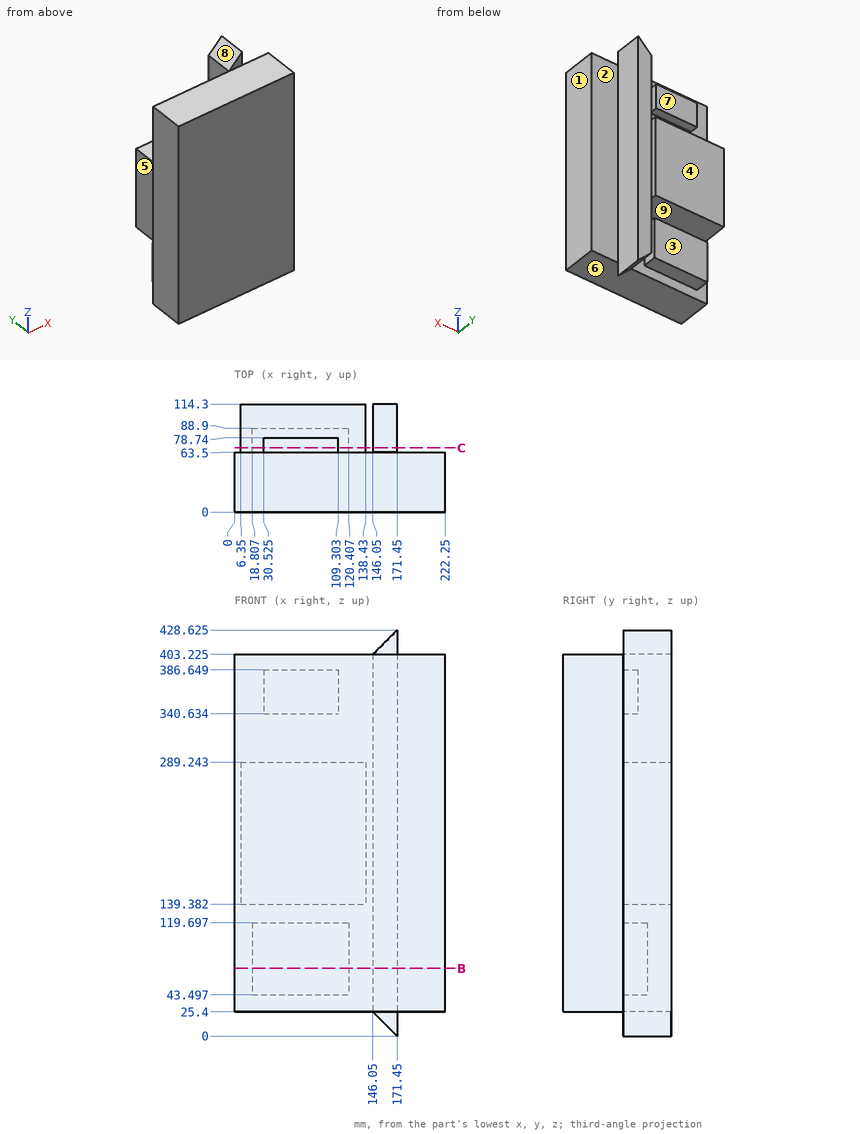
Geometry check sheet. Reference: drawing and pictorial views, mm from the part's lowest x, y, z. A direction names the side the tool comes from. Round coordinates to 2 decimals unless told otherwise and drop trailing zeros. Write each loop counter-clockwise with the first axis right and the second up, starting at its lowest first coordinate (ties: lowest second). Pieces come first, ordered by that corner, then holes. Notation, with made-up numbers: (19.5, -8.75) -> (58.5, -8.75) arc R20 cw to (58.5, 16.25) -> close; hole circle Ø1 at (46, -26). An arc over 180 degrees is marked (long way). Put each result on its own line as item: value.
1) Depth check by flat-ended pin: P1, Ø1.5, axis at x = 193, z = 345, coming from the +Y side; P2, Ø12, axis at x = 70.5, y = 74.5, coming from the +Z side; P3, Ø4.5, axis at y = 67.5, z = 365.5, coming from the -X side (1 decimal). Enter the tip coordinate at first touch or a pass-through.
Recorded:
P1: stops at y = 63.5
P2: stops at z = 386.65
P3: stops at x = 30.5
2) Cross-section at B-B, the plane z = 71.5. Enter the section's corners in (x, y).
Recorded:
outline: (0, 0) -> (222.25, 0) -> (222.25, 63.5) -> (171.45, 63.5) -> (171.45, 114.3) -> (146.05, 114.3) -> (146.05, 63.5) -> (120.41, 63.5) -> (120.41, 88.9) -> (18.81, 88.9) -> (18.81, 63.5) -> (0, 63.5) -> close
3) Cross-section at C-C, the plane y = 68. Give the number of separate pieces and of enclosed holes in the cut face, plus the area to 3 significant figures.
Recorded:
separate pieces: 4
enclosed holes: 0
area: 41,400 mm2
4) Release check for a two-part mould opening along Z. For the marked faces 6, 7, 8 and 9 record: pulls with the +Z half, pulls with the -Z half, needs draft (parallel to the pull), parting line crosses it, or undercut.
Recorded:
face 6: pulls with the -Z half
face 7: needs draft
face 8: pulls with the +Z half
face 9: undercut
5) Access from +Z, -Z, +X, -X, +Y, -Y to the whole of each face (thin tool, end or side, straight path). Record for the marked faces 1, 2, 3, 4 and 5.
Recorded:
face 1: +Z, -Z, +X, +Y, -Y
face 2: +Z, -Z, +X, +Y
face 3: -Z, -X, +Y
face 4: +Z, -Z, +X, -X, +Y
face 5: +Z, -Z, -X, +Y
6) Thickness scan on probe 1 along X at (y, z) = (86, 263); probe 2 along Z at (x, y) = (51, 67); probe 3 along Z at (x, y) = (62, 99.5). Record the ranges inside material, lowest first. Write a range as from..to.
Recorded:
probe 1: x = 6.35..138.43, 146.05..171.45
probe 2: z = 43.5..119.7, 139.38..289.24, 340.63..386.65
probe 3: z = 139.38..289.24
